Can you work these out from the model? Positions are in its coordinate system, mm. A direction names the side the tool comes from. Round coordinates to 2 decimals unless told otherwise and drop trailing zeros. Write each loop counter-clockwise with the first axis right and the second up, starting at its lowest first coordinate (ties: lowest second). Pieces come first, ordered by that corner, then holes. Notation, with made-up numbers: (-35.75, 22) -> (-12.75, 22) arc R25 ccw to (-12.75, 55) -> close; hole circle Ø9 at (63.25, 66). An arc over 180 degrees is marked (long way). Write item = value, one per line. Start each with the question number.
1) Imagine slicing it at A-A, the plane x = 0. Please give me the cut outline in (y, z).
2) If I drill on line 1 (Z direction, x = 2.75, y = 0.2); line 2 (Z direction, x = 0.5, y = 0.9); line 3 (X direction, y = 0.8, z = 3.5), over which ranges is the centre line in solid material (lowest first)?
3) I'm going to push flat-ended pins straight in: pin 1 (1.8 mm diameter, centred on x = 1, y = 1.5, fed in from +Z); pin 2 (2 mm diameter, centred on x = 1, y = 0.5, fed in from +Z); pin 3 (1.5 mm diameter, centred on x = -3, z = 10, fed in from +Y). Where does each tip first touch, or does it pass through?
4) Imagine slicing it at C-C, the plane z = 3.75. Please give me the cut outline in (x, y), then the cut area to 3 significant figures.
5) Thinking about a two-plate mould opening in X: for faces 1 (the face through (0.078, 3.555, 8.284)), 2 (the face through (2.3, 0, 5.5)), 3 (the face through (0.039, 1.778, 3.37)), which applies, +X half, -X half, draft (parallel to the pull), parting line (faces both ways), or undercut?
6) Imagine slicing it at B-B, the plane z = 6. Please give me the cut outline in (x, y) (1 decimal), then the cut area to 3 significant figures.
7) For faces 4 (the face through (0.06, 2.92, 11.4)), 5 (the face through (0.07, 3.16, 0.96)), which set-ups out of +Z, -Z, +X, -X, +Y, -Y let a thin tool reach every point of the face, with its end or its side?
from build123d import *

# Parameters (mm, degrees)
F1_ANGLE = 180


with BuildPart() as f1:
    # F0 (on Front) → F1 (revolve)
    with BuildSketch(Plane.XZ):
        Polygon((2.904469, 0), (3.556, 2.431545), (3.556, 13.974021), (2.921, 13.974021), (2.921, 8.894021), (2.2225, 8.894021), (2.2225, 5.7912), (1.778, 5.7912), (1.778, 1.016), (0, 1.016), (0, 0), align=None)
    revolve(axis=Axis((0, 0, 0.508), (0, 0, 1)), revolution_arc=F1_ANGLE)


solid = f1.part
Reported:
q1.outline = (0, 0) -> (2.9, 0) -> (3.56, 2.43) -> (3.56, 13.97) -> (2.92, 13.97) -> (2.92, 8.89) -> (2.22, 8.89) -> (2.22, 5.79) -> (1.78, 5.79) -> (1.78, 1.02) -> (0, 1.02) -> close
q2.line_1 = 0 to 8.89
q2.line_2 = 0 to 1.02
q2.line_3 = -3.46 to -1.59, 1.59 to 3.46
q3.pin_1 = 8.89
q3.pin_2 = 5.79
q3.pin_3 = 2.75
q4.outline = (-3.56, 0) -> (-1.78, 0) arc R1.78 cw to (1.78, 0) -> (3.56, 0) arc R3.56 ccw to start
q4.area = 14.9 mm²
q5.face_1 = parting line
q5.face_2 = draft
q5.face_3 = undercut
q6.outline = (-3.6, 0) -> (-2.2, 0) arc R2.2 cw to (2.2, 0) -> (3.6, 0) arc R3.6 ccw to start
q6.area = 12.1 mm²
q7.face_4 = +Z, -Y
q7.face_5 = -Z, +Y
